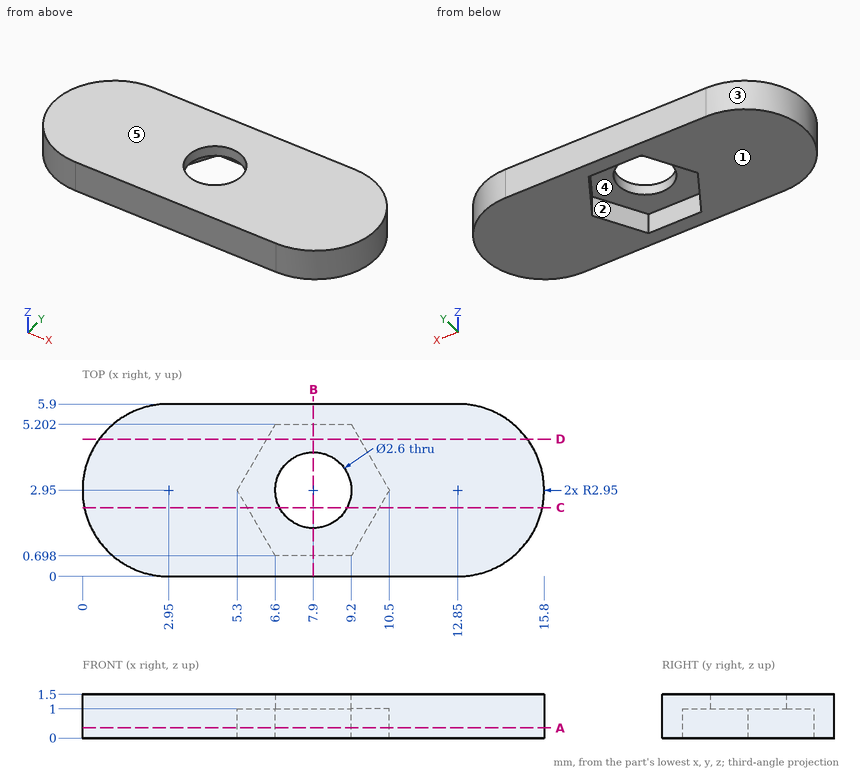
Geometry: see drawing. Coordinates: mm, zero at the bounding-box minimum. A direction names the side the tool comes from. Round coordinates to 2 decimals unless told otherwise and drop trailing zeros. Write each loop counter-clockwise with the first axis right and the second up, starting at its lowest first coordinate (ties: lowest second). Pieces come first, ordered by that corner, then holes.
Item 1: Material intervals for L1, parallel to Y at x = 7.9, z = 1.4; L2, parallel to X at y = 2.9, z = 1.35; L3, parallel to X at y = 3.7, z = 1.1, sorted ascending.
Item 2: Section query C-C (y = 2.35). Return loops of the section in (x, z).
Item 3: Set-up query: the marked faces 1 and 2. Return all of +Z, -Z, +X, -X, +Y, -Y with unobstructed straight access to the full face (end or side cutting, diameter ignored); none if empty.
Item 4: Section query B-B (x = 7.9). Return loops of the section in (y, z).
Item 5: Mould query, pull axis Y, two halves, no side actions, for the marked faces 3, 4 and 5. Classes: +Y half, -Y half, draft (parallel to the pull), parting line (faces both ways), or undercut.
Item 6: Pin query (flat end, axial travel): P1, Ø1.5, axis at x = 7.5, y = 2, coming from the -Z side. Return the tip coordinate at first contact, or that it passes through.
Item 7: Section query A-A (z = 0.35). Return loops of the section in (x, y).
Item 8: Section query D-D (y = 4.7). Return loops of the section in (x, z) (1 decimal), plus the area to 3 significant figures.
Completed:
1. L1: y = 0 to 1.65, 4.25 to 5.9
1. L2: x = 0 to 6.6, 9.2 to 15.8
1. L3: x = 0.1 to 6.84, 8.96 to 15.7
2. outline: (0.06, 0) - (5.65, 0) - (5.65, 1) - (6.75, 1) - (6.75, 1.5) - (0.06, 1.5) - close; (9.05, 1) - (10.15, 1) - (10.15, 0) - (15.74, 0) - (15.74, 1.5) - (9.05, 1.5) - close
3. face 1: -Z, +X, -X, +Y, -Y
3. face 2: -Z
4. outline: (0, 0) - (0.7, 0) - (0.7, 1) - (1.65, 1) - (1.65, 1.5) - (0, 1.5) - close; (4.25, 1) - (5.2, 1) - (5.2, 0) - (5.9, 0) - (5.9, 1.5) - (4.25, 1.5) - close
5. face 3: parting line
5. face 4: undercut
5. face 5: draft
6. P1: stops at z = 1
7. outline: (2.95, 0) - (12.85, 0) arc R2.95 ccw to (12.85, 5.9) - (2.95, 5.9) arc R2.95 ccw to start; hole (5.3, 2.95) - (6.6, 0.7) - (9.2, 0.7) - (10.5, 2.95) - (9.2, 5.2) - (6.6, 5.2) - close
8. outline: (0.6, 0) - (6.3, 0) - (6.3, 1) - (9.5, 1) - (9.5, 0) - (15.2, 0) - (15.2, 1.5) - (0.6, 1.5) - close
8. area: 18.8 mm2
